The listing builds one solid part. Answer for the finished solid, in the listing's coordinates (mm). Face numbers are marked on the shaded views. A direction names the side the tool comes from. Round coordinates to 2 decimals unless told otherwise and drop trailing zeros. Order: outer loops, then holes, each group sorted by start corner. A loop starts at its lowest first (then second) coordinate and runs counter-clockwise, first axis right, second up. Notation, with made-up numbers: M 24.5,65.25 L 54.5,65.25 A31 ccw 54.5,103.25 Z; hole C -3,84.25 d5. An arc over 180 degrees is marked long. Put each result on its own line as item: value. Start each with the question number.
1. The part is cut by section C-C (z = 52). Give the vertices of the cut face in (x, y), then the cut area to 3 significant figures.
2. Each of these flat-tipped pins is pushed along its axis until it touches: pin 1 Ø6.5 at (y, z) = (95.5, -1.5) entering from +X; pin 2 Ø18 at (y, z) = (98.5, 5.5) entering from -X; pin 3 Ø5.5 at (x, z) = (41.28, 52.39) entering from -Y; pin 4 Ø7.5 at (x, z) = (-41.28, -52.39) entering from -Y. Where does it stop, or does it pass through?
3. The part is cut by section B-B (y = 96). Give the vertices of the cut face in (x, z).
4. Which of the six approach directions +Z, -Z, +X, -X, +Y, -Y give full straight-line access (tool end or side, diameter ignored) to the marked faces 1, 2, 3 and 4?
5. Consider line 1 (Z direction, x = 40, y = 1.5); line 2 (X direction, y = 71, z = 54.5); line 3 (X direction, y = 102, z = 23). Determine where each line is inside the solid, lowest interval first.
6. The part is cut by section A-A (z = 27). Give the vertices of the cut face in (x, y) (3 decimals), then the cut area to 3 significant figures.
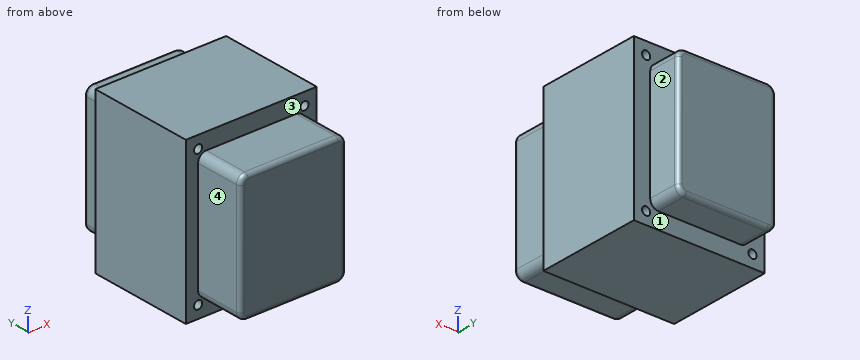
Autodesk Inventor part; units mm, degrees
ref_plane "YZ Plane" through (0, 0, 0) normal (1, 0, 0) x (0, 1, 0)
ref_plane "XZ Plane" through (0, 0, 0) normal (0, 1, 0) x (-1, 0, 0)
ref_plane "XY Plane" through (0, 0, 0) normal (0, 0, 1) x (1, 0, 0)
sketch "Sketch1" plane through (0, 0, 0) normal (0, 1, 0) x (-1, 0, 0)
  line L0 (-50.8, 61.9125) -> (50.8, 61.9125)
  line L1 (50.8, 61.9125) -> (50.8, -61.9125)
  line L2 (50.8, -61.9125) -> (-50.8, -61.9125)
  line L3 (-50.8, -61.9125) -> (-50.8, 61.9125)
  line L4 (-50.8, 61.9125) -> (50.8, -61.9125) construction
  line L5 (50.8, 61.9125) -> (-50.8, -61.9125) construction
  point P0 (0, 0)
  dimension "d0" = 123.825
  dimension "d1" = 101.6
extrude "Extrusion1" add sketch "Sketch1" along normal blind 82.55
sketch "Sketch2" plane through (0, 82.55, 0) normal (0, 1, 0) x (1, 0, 0)
  line L0 (31.75, -49.2125) -> (-31.75, -49.2125)
  line L1 (-38.1, -42.8625) -> (-38.1, 42.8625)
  line L2 (-31.75, 49.2125) -> (31.75, 49.2125)
  line L3 (38.1, 42.8625) -> (38.1, -42.8625)
  line L4 (38.1, -49.2125) -> (-38.1, 49.2125) construction
  line L5 (-38.1, -49.2125) -> (38.1, 49.2125) construction
  arc A0 (-38.1, -42.8625) -> (-31.75, -49.2125) centre (-31.75, -42.8625) ccw
  arc A1 (-31.75, 49.2125) -> (-38.1, 42.8625) centre (-31.75, 42.8625) ccw
  arc A2 (38.1, 42.8625) -> (31.75, 49.2125) centre (31.75, 42.8625) ccw
  arc A3 (31.75, -49.2125) -> (38.1, -42.8625) centre (31.75, -42.8625) ccw
  line L6 (-50.8, 61.9125) -> (-50.8, -61.9125)
  line L7 (50.8, 61.9125) -> (-50.8, 61.9125)
  point P0 (0, 0)
  dimension "d6" = 6.35
  dimension "d25" = 12.7
  dimension "d26" = 12.7
extrude "Extrusion2" add sketch "Sketch2" along normal blind 25.4
fillet "Fillet1" radius 3.175 8 edges at (36.2401, 107.95, 47.3526) (38.1, 107.95, 0) (36.2401, 107.95, -47.3526) (0, 107.95, -49.2125) (-36.2401, 107.95, -47.3526) (-38.1, 107.95, 0) (-36.2401, 107.95, 47.3526) (0, 107.95, 49.2125)
hole "Hole1" at (41.275, 82.55, 52.3875) direction (0, -1, 0) diameter 6.35 end through all
pattern_linear "Rectangular Pattern1" count 2 spacing 104.775 along (0, 0, -1) count 2 spacing 82.55 along (-1, 0, 0) of "Hole1"
sketch "Sketch3" plane through (0, 0, 0) normal (0, -1, 0) x (1, 0, 0)
  line L0 (-34.925, -49.2125) -> (34.925, -49.2125)
  line L1 (41.275, -42.8625) -> (41.275, 42.8625)
  line L2 (34.925, 49.2125) -> (-34.925, 49.2125)
  line L3 (-41.275, 42.8625) -> (-41.275, -42.8625)
  line L4 (-41.275, -49.2125) -> (41.275, 49.2125) construction
  line L5 (41.275, -49.2125) -> (-41.275, 49.2125) construction
  line L6 (50.8, 61.9125) -> (-50.8, 61.9125)
  line L7 (50.8, -61.9125) -> (50.8, 61.9125)
  arc A0 (-34.925, 49.2125) -> (-41.275, 42.8625) centre (-34.925, 42.8625) ccw
  arc A1 (41.275, 42.8625) -> (34.925, 49.2125) centre (34.925, 42.8625) ccw
  arc A2 (34.925, -49.2125) -> (41.275, -42.8625) centre (34.925, -42.8625) ccw
  arc A3 (-41.275, -42.8625) -> (-34.925, -49.2125) centre (-34.925, -42.8625) ccw
  point P0 (0, 0)
  dimension "d27" = 12.7
  dimension "d28" = 9.525
  dimension "d29" = 6.35
extrude "Extrusion3" add sketch "Sketch3" along normal blind 38.1
fillet "Fillet2" radius 3.175 8 edges at (-39.4151, -38.1, 47.3526) (-41.275, -38.1, 0) (-39.4151, -38.1, -47.3526) (0, -38.1, -49.2125) (39.4151, -38.1, -47.3526) (41.275, -38.1, 0) (39.4151, -38.1, 47.3526) (0, -38.1, 49.2125)
properties part number "xmfr power"
Resolved:
1. outline: M -50.8,0 L -44.43,0 L -44.43,82.55 L -50.8,82.55 Z; M -38.12,0 L 38.12,0 L 38.12,82.55 L -38.12,82.55 Z; M 44.43,0 L 50.8,0 L 50.8,82.55 L 44.43,82.55 Z
1. area: 7,350 mm2
2. pin 1: x = 38.1
2. pin 2: x = -38.1
2. pin 3: through
2. pin 4: y = 0
3. outline: M -38.1,-42.86 A6.35 ccw -31.75,-49.21 L 31.75,-49.21 A6.35 ccw 38.1,-42.86 L 38.1,42.86 A6.35 ccw 31.75,49.21 L -31.75,49.21 A6.35 ccw -38.1,42.86 Z
4. face 1: +Y
4. face 2: +Z, -Z, +X, +Y
4. face 3: -Y
4. face 4: +Z, -Z, -X, -Y
5. line 1: -61.91 to -55.3, -49.48 to 49.48, 55.3 to 61.91
5. line 2: -50.8 to -43.65, -38.9 to 38.9, 43.65 to 50.8
5. line 3: -38.1 to 38.1
6. outline: M -50.8,0 L -41.275,0 L -41.275,-34.925 A3.175 ccw -38.1,-38.1 L 38.1,-38.1 A3.175 ccw 41.275,-34.925 L 41.275,0 L 50.8,0 L 50.8,82.55 L 38.1,82.55 L 38.1,104.775 A3.175 ccw 34.925,107.95 L -34.925,107.95 A3.175 ccw -38.1,104.775 L -38.1,82.55 L -50.8,82.55 Z
6. area: 13,500 mm2
